from build123d import *

# Parameters (mm, degrees)
BOSS_EXTRUDE1_DEPTH = 25
CUT_EXTRUDE2_DEPTH  = 26
BOSS_EXTRUDE2_DEPTH = 0.4


with BuildPart() as part:
    # Sketch1 → Boss-Extrude1 (new body)
    with BuildSketch(Plane(origin=(0, 0, 0), x_dir=(1, 0, 0), z_dir=(0, 1, 0))):
        with BuildLine():
            ThreePointArc((1.451818925, -34.068556857), (1.641248992, -34.346908706), (1.964225605, -34.442038138))
            ThreePointArc((1.964225605, -34.442038138), (26.591847487, -21.978073076), (34.198225299, 4.555174015))
            ThreePointArc((34.198225299, 4.555174015), (23.590291339, 25.176355888), (2.324135821, 34.423627607))
            ThreePointArc((2.324135821, 34.423627607), (1.751838249, 34.289058819), (1.354061739, 33.856153382))
            ThreePointArc((1.354061739, 33.856153382), (0, 33.001534515), (-1.354061739, 33.856153382))
            ThreePointArc((-1.354061739, 33.856153382), (-1.751838249, 34.289058819), (-2.324135821, 34.423627607))
            ThreePointArc((-2.324135821, 34.423627607), (-23.590291339, 25.176355888), (-34.198225299, 4.555174015))
            ThreePointArc((-34.198225299, 4.555174015), (-26.591847487, -21.978073076), (-1.964225605, -34.442038138))
            ThreePointArc((-1.964225605, -34.442038138), (-1.641248992, -34.346908706), (-1.451818925, -34.068556857))
            ThreePointArc((-1.451818925, -34.068556857), (0, -32.945679925), (1.451818925, -34.068556857))
        make_face()
        with BuildLine():
            Line((-2.417, 3.787737139), (0, 3.787737139))
            Line((0, 3.787737139), (2.417, 3.787737139))
            ThreePointArc((2.417, 3.787737139), (0, -4.489512172), (-2.417, 3.787737139))
        make_face(mode=Mode.SUBTRACT)
    extrude(amount=BOSS_EXTRUDE1_DEPTH)

    # Sketch2 → Cut-Extrude2 (cut, through all)
    with BuildSketch(Plane(origin=(0, 0, 0), x_dir=(1, 0, 0), z_dir=(0, 1, 0))):
        with BuildLine():
            ThreePointArc((-32.364754098, -2.961873082), (-22.980970389, -22.980970389), (-2.961873082, -32.364754098))
            ThreePointArc((-2.961873082, -32.364754098), (-1.976534873, -32.204764677), (-1.191258844, -31.588461538))
            ThreePointArc((-1.191258844, -31.588461538), (0, -31), (1.191258844, -31.588461538))
            ThreePointArc((1.191258844, -31.588461538), (1.976534873, -32.204764677), (2.961873082, -32.364754098))
            ThreePointArc((2.961873082, -32.364754098), (22.980970389, -22.980970389), (32.364754098, -2.961873082))
            ThreePointArc((32.364754098, -2.961873082), (32.204764677, -1.976534873), (31.588461538, -1.191258844))
            ThreePointArc((31.588461538, -1.191258844), (31, 0), (31.588461538, 1.191258844))
            ThreePointArc((31.588461538, 1.191258844), (32.204764677, 1.976534873), (32.364754098, 2.961873082))
            ThreePointArc((32.364754098, 2.961873082), (22.980970389, 22.980970389), (2.961873082, 32.364754098))
            ThreePointArc((2.961873082, 32.364754098), (1.976534873, 32.204764677), (1.191258844, 31.588461538))
            ThreePointArc((1.191258844, 31.588461538), (0, 31), (-1.191258844, 31.588461538))
            ThreePointArc((-1.191258844, 31.588461538), (-1.976534873, 32.204764677), (-2.961873082, 32.364754098))
            ThreePointArc((-2.961873082, 32.364754098), (-22.980970389, 22.980970389), (-32.364754098, 2.961873082))
            ThreePointArc((-32.364754098, 2.961873082), (-32.204764677, 1.976534873), (-31.588461538, 1.191258844))
            ThreePointArc((-31.588461538, 1.191258844), (-31, 0), (-31.588461538, -1.191258844))
            ThreePointArc((-31.588461538, -1.191258844), (-32.204764677, -1.976534873), (-32.364754098, -2.961873082))
        make_face()
    extrude(amount=CUT_EXTRUDE2_DEPTH, mode=Mode.SUBTRACT)

    # Sketch2<2> → Boss-Extrude2 (add)
    with BuildSketch(Plane(origin=(0, 0, 0), x_dir=(1, 0, 0), z_dir=(0, 1, 0))):
        with BuildLine():
            ThreePointArc((-32.364754098, -2.961873082), (-22.980970389, -22.980970389), (-2.961873082, -32.364754098))
            ThreePointArc((-2.961873082, -32.364754098), (-1.976534873, -32.204764677), (-1.191258844, -31.588461538))
            ThreePointArc((-1.191258844, -31.588461538), (0, -31), (1.191258844, -31.588461538))
            ThreePointArc((1.191258844, -31.588461538), (1.976534873, -32.204764677), (2.961873082, -32.364754098))
            ThreePointArc((2.961873082, -32.364754098), (22.980970389, -22.980970389), (32.364754098, -2.961873082))
            ThreePointArc((32.364754098, -2.961873082), (32.204764677, -1.976534873), (31.588461538, -1.191258844))
            ThreePointArc((31.588461538, -1.191258844), (31, 0), (31.588461538, 1.191258844))
            ThreePointArc((31.588461538, 1.191258844), (32.204764677, 1.976534873), (32.364754098, 2.961873082))
            ThreePointArc((32.364754098, 2.961873082), (22.980970389, 22.980970389), (2.961873082, 32.364754098))
            ThreePointArc((2.961873082, 32.364754098), (1.976534873, 32.204764677), (1.191258844, 31.588461538))
            ThreePointArc((1.191258844, 31.588461538), (0, 31), (-1.191258844, 31.588461538))
            ThreePointArc((-1.191258844, 31.588461538), (-1.976534873, 32.204764677), (-2.961873082, 32.364754098))
            ThreePointArc((-2.961873082, 32.364754098), (-22.980970389, 22.980970389), (-32.364754098, 2.961873082))
            ThreePointArc((-32.364754098, 2.961873082), (-32.204764677, 1.976534873), (-31.588461538, 1.191258844))
            ThreePointArc((-31.588461538, 1.191258844), (-31, 0), (-31.588461538, -1.191258844))
            ThreePointArc((-31.588461538, -1.191258844), (-32.204764677, -1.976534873), (-32.364754098, -2.961873082))
        make_face()
    extrude(amount=BOSS_EXTRUDE2_DEPTH)


solid = part.part
Input: part model. Units: mm. Frame: model coordinates. A direction names the side the tool comes from. Coordinates: 2 decimals unless noted, no trailing zeros. Order: outer loops, then holes, each group sorted by start corner. A loop starts at its lowest first (then second) coordinate and runs counter-clockwise, first axis right, second up.
1. Draft query along Z for faces 3 (the flat face through (0, 0, 0)), 4 (the cylindrical face through (-32.199, 12.528, 1.964)), 5 (the cylindrical face through (0, 12, -33)). Return one class per face: +Z half, -Z half, draft (parallel to the pull), parting line (faces both ways), or undercut.
Checked values:
face 3: draft
face 4: undercut
face 5: -Z half
2. Cut plane C-C, the plane z = -12. Return loops of the section in (x, y), plus the area to 3 significant figures.
Checked values:
outline: (-32.35, 0) - (32.35, 0) - (32.35, 25) - (30.2, 25) - (30.2, 0.4) - (-30.2, 0.4) - (-30.2, 25) - (-32.35, 25) - close
area: 131 mm2
3. Cut plane A-A, the plane y = 13.5. Return loops of the section in (x, z).
Checked values:
outline: (-2.32, -34.42) arc R1 ccw to (-1.35, -33.86) arc R1.5 cw to (1.35, -33.86) arc R1 ccw to (2.32, -34.42) arc R34.5 ccw to (1.96, 34.44) arc R0.5 ccw to (1.45, 34.07) arc R1.5 cw to (-1.45, 34.07) arc R0.5 ccw to (-1.96, 34.44) arc R34.5 ccw to start; hole (-32.36, -2.96) arc R32.5 ccw to (-2.96, -32.36) arc R2 ccw to (-1.19, -31.59) arc R1.5 cw to (1.19, -31.59) arc R2 ccw to (2.96, -32.36) arc R32.5 ccw to (32.36, -2.96) arc R2 ccw to (31.59, -1.19) arc R1.5 cw to (31.59, 1.19) arc R2 ccw to (32.36, 2.96) arc R32.5 ccw to (2.96, 32.36) arc R2 ccw to (1.19, 31.59) arc R1.5 cw to (-1.19, 31.59) arc R2 ccw to (-2.96, 32.36) arc R32.5 ccw to (-32.36, 2.96) arc R2 ccw to (-31.59, 1.19) arc R1.5 cw to (-31.59, -1.19) arc R2 ccw to start
4. Cut plane B-B, the plane x = -27.5. Return loops of the section in (y, z), plus the area to 3 significant figures.
Checked values:
outline: (0, -20.83) - (25, -20.83) - (25, -17.32) - (0.4, -17.32) - (0.4, 17.32) - (25, 17.32) - (25, 20.83) - (0, 20.83) - close
area: 189 mm2
5. Contact query for flat-ended pins moving along their axis: P1, Ø4, axis at x = 26.5, z = 11, coming from the +Y side; P2, Ø12, axis at y = 13, z = -3.5, coming from the -X side; P3, Ø5, axis at x = -27.5, y = 6.5, coming from the -Z side. Output: stop coordinate, or through.
Checked values:
P1: stops at y = 0.4
P2: stops at x = -34.5
P3: stops at z = -23.78
6. Ray query, line 1 along Y through (x, z) = (-10, 28.5); line 2 along X through (y, z) = (24, -8.5); line 3 along Z through (x, y) = (15.5, 10.75). Return the intervals inside material, ascending.
Checked values:
line 1: y = 0 to 0.4
line 2: x = -33.44 to -31.37, 31.37 to 33.44
line 3: z = -30.82 to -28.57, 28.57 to 30.82
7. Access query for faces 1 (the cylindrical face through (31, 13, 0)), 2 (the cylindrical face through (-0.028, 12.325, 32.946)). Directions: +Z, -Z, +X, -X, +Y, -Y. A direction counts if a zero-diameter tool reaches every point of the face in a straight line with its end or side. Return the directions, or none.
Checked values:
face 1: +Y
face 2: +Z, +Y, -Y
